Build history of the part. All positions in model axes, mm. A direction names the side the tool comes from. Round coordinates to 2 decimals unless told otherwise and drop trailing zeros. Order: outer loops, then holes, each group sorted by start corner. A loop starts at its lowest first (then second) coordinate and runs counter-clockwise, first axis right, second up. Notation, with made-up numbers: (34, -19) -> (59, -19) arc R30 ccw to (59, 11) -> close; hole circle Ø3 at (27, 34). An arc over 180 degrees is marked (long way). Use a Markdown table: item, result. Add a question column.
Item 1: 3-axis set-ups, long thin cutter, end or side, ignore diameter. For faces 5 (the face through (0, 18, 20)), 6 (the face through (-5, 0, 24)), 7 (the face through (6.154, 4.957, -9.349)): which of +Z, -Z, +X, -X, +Y, -Y reach the whole face in a straight line?
Item 2: Pin check, flat tips, straight feed: pin 1 (1.5 mm diameter, centred on y = 6, z = -21, fed in from -X); pin 2 (3 mm diameter, centred on x = -14.5, z = 19.5, fed in from -Y); pin 3 (3 mm diameter, centred on y = -6.5, z = -4, fed in from -X); pin 4 (8 mm diameter, centred on y = 4, z = -17.5, fed in from -X). Stop position of each tip, or through.
Item 3: Slice it at C-C, the plane x = 0. Give the cut face in (y, z), plus the area to 3 significant figures.
Item 4: Slice it at B-B, the plane z = -10. Give the cut face in (x, y), plus the area to 3 significant figures.
Item 5: Slice it at D-D, the plane x = 14.5. Give the cut face in (y, z), plus the area to 3 significant figures.
Item 6: Probe L1, parallel to Z at x = 6.25, y = 0; L2, parallel to Y at x = 0.5, z = -10; L3, parallel to Z at x = 2, y = 17. List the from-to ranges inside material, lowest first.
Item 7: Two-plate mould, pull along X, no slides. Class faces 1 (the face through (-4.336, -19.524, 0.49)), 2 (the face through (16.77, 1.5, 0.21)), 3 (the face through (-5, 0, -23)), 4 (the face through (0, 18, -20)): released by +X, released by -X, zero draft, split by the parting line, or undercut.
Item 8: Slice it at A-A, the plane y = 0. Give the cut face in (x, z).
from build123d import *

# Parameters (mm, degrees)
SKETCH1_R               = 20
BOSS_EXTRUDE1_DEPTH     = 35
SKETCH3_R               = 5
SKETCH4_W               = 40
SKETCH4_H               = 4
CUT_EXTRUDE1_DEPTH      = 21
CUT_EXTRUDE1_DEPTH_BACK = 21


with BuildPart() as part:
    # Sketch1 → Boss-Extrude1 (new body, symmetric)
    with BuildSketch(Plane.XY):
        Circle(SKETCH1_R)
    extrude(amount=BOSS_EXTRUDE1_DEPTH, both=True)

    # Cut-Sweep1: sweep along a path in Sketch2
    with BuildLine(Plane(origin=(0, 0, 0), x_dir=(1, 0, 0), z_dir=(0, 1, 0))) as cut_sweep1_path:
        Line((0, 35), (0, 10))
        Line((0, 10), (12, 10))
        Line((12, 10), (12, -10))
        Line((12, -10), (0, -10))
        Line((0, -10), (0, -35))
    # Sketch3 → Cut-Sweep1 (sweep, cut)
    with BuildSketch(Plane.XY.offset(35)):
        Circle(SKETCH3_R)
    sweep(path=cut_sweep1_path.line, transition=Transition.RIGHT, mode=Mode.SUBTRACT)

    # Sketch4 → Cut-Extrude1 (cut, two sides)
    with BuildSketch(Plane(origin=(0, 0, 0), x_dir=(0, 0, -1), z_dir=(1, 0, 0))) as cut_extrude1_sk:
        with Locations((0, 18)):
            Rectangle(SKETCH4_W, SKETCH4_H)
    extrude(amount=CUT_EXTRUDE1_DEPTH, mode=Mode.SUBTRACT)
    extrude(cut_extrude1_sk.sketch, amount=-CUT_EXTRUDE1_DEPTH_BACK, mode=Mode.SUBTRACT)


solid = part.part
Check sheet entries:
| question | item | result |
|---|---|---|
| 1 | face 5 | +X, -X, +Y |
| 1 | face 6 | +Z |
| 1 | face 7 | none |
| 2 | pin 1 | x = -19.3 |
| 2 | pin 2 | y = -15.2 |
| 2 | pin 3 | x = -19.36 |
| 2 | pin 4 | x = -20 |
| 3 | outline | (-20, -35) -> (-5, -35) -> (-5, -10) arc R5 cw to (5, -10) -> (5, -35) -> (20, -35) -> (20, -20) -> (16, -20) -> (16, 20) -> (20, 20) -> (20, 35) -> (5, 35) -> (5, 10) arc R5 cw to (-5, 10) -> (-5, 35) -> (-20, 35) -> close |
| 3 | area | 2,060 mm2 |
| 4 | outline | (-12, 16) arc R20 ccw (long way) to (12, 16) -> close; hole (0, -5) -> (12, -5) arc R5 ccw to (12, 5) -> (0, 5) arc R5 ccw to start |
| 4 | area | 993 mm2 |
| 5 | outline | (-13.77, -35) -> (13.77, -35) -> (13.77, 35) -> (-13.77, 35) -> close; hole (-4.33, -12.5) arc R5 ccw to (4.33, -12.5) -> (4.33, 12.5) arc R5 ccw to (-4.33, 12.5) -> close |
| 5 | area | 1,680 mm2 |
| 6 | L1 | -35 to -15, -5 to 5, 15 to 35 |
| 6 | L2 | -19.99 to -5, 5 to 16 |
| 6 | L3 | -35 to -20, 20 to 35 |
| 7 | face 1 | split by the parting line |
| 7 | face 2 | undercut |
| 7 | face 3 | undercut |
| 7 | face 4 | zero draft |
| 8 | outline | (-20, -35) -> (-5, -35) -> (-5, -5) -> (7, -5) -> (7, 5) -> (-5, 5) -> (-5, 35) -> (-20, 35) -> close; (5, -35) -> (20, -35) -> (20, 35) -> (5, 35) -> (5, 15) -> (17, 15) -> (17, -15) -> (5, -15) -> close |
